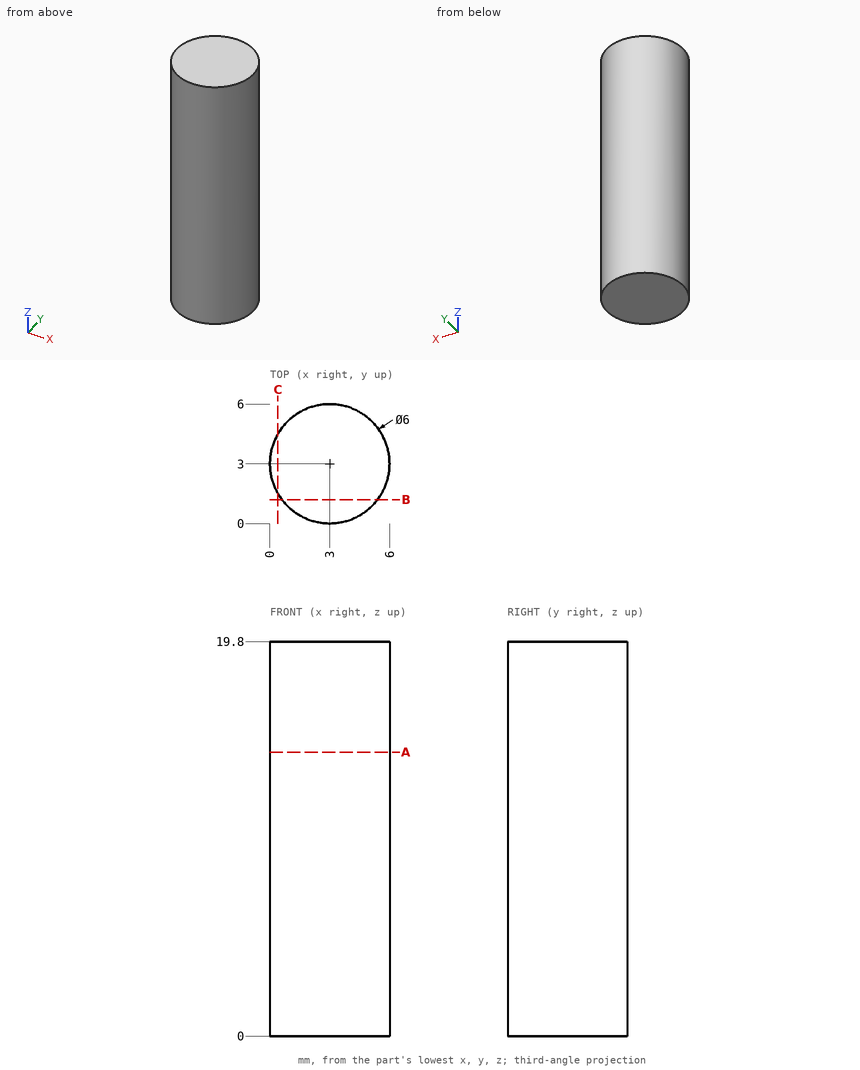
Design review of the part shown in the three views and the two pictorial views. Dimensions are in mm from the part's minimum x, y and z. Round coordinates to 2 decimals unless told otherwise and drop trailing zeros. Loops run counter-clockwise (first coordinate to the right, second up) from the corner with the lowest first, then second, coordinate; pieces in that order, holes last. Notation, with made-up numbers: (59.5, 63.25) - (97.5, 63.25) arc R15 cw to (97.5, 88.25) - close; hole circle Ø4 at (76, 38). An arc over 180 degrees is marked (long way). Use one line per item in the form item = value.
1) Clearance check with a flat-ended pin moving along its axis: P1, Ø3, axis at y = 5, z = 16.5, coming from the +X side. State where the tip first meets the part, or that it passes through.
Solutions:
P1 = 5.96
2) Wall thickness on probe 1 along X at (y, z) = (3.75, 16.75); probe 2 along Y at (x, z) = (2.6, 5.5); probe 3 along X at (y, z) = (4.5, 3): over which ranges is each line inside the solid? List them lowest first.
Solutions:
probe_1 = 0.1 to 5.9
probe_2 = 0.03 to 5.97
probe_3 = 0.4 to 5.6
3) We need section C-C on x = 0.4. Write out the cut boundary in (y, z), then the cut area to 3 significant figures.
Solutions:
outline = (1.5, 0) - (4.5, 0) - (4.5, 19.8) - (1.5, 19.8) - close
area = 59.3 mm2
4) We need section B-B on y = 1.2. Write out the cut boundary in (x, z).
Solutions:
outline = (0.6, 0) - (5.4, 0) - (5.4, 19.8) - (0.6, 19.8) - close
5) We need section A-A on z = 14.25. Write out the cut boundary in (x, y), then the cut area to 3 significant figures.
Solutions:
outline = circle Ø6 at (3, 3)
area = 28.3 mm2
